```python
from build123d import *

# Parameters (mm, degrees)
F0_W      = 14.8
F0_H      = 16.7
F0_W_2    = 11.8
F0_H_2    = 13.7
F1_DEPTH  = 11.95
F2_W      = 12.65
F2_H      = 16.7
F2_W_2    = 10.65
F2_H_2    = 14.7
F3_DEPTH  = 7
F4_W      = 0.575
F4_H      = 13.7
F5_DEPTH  = 11.95
F6_W      = 0.575
F6_H      = 13.7
F7_DEPTH  = 11.95
F8_W      = 10.65
F8_H      = 0.5
F9_DEPTH  = 7
F10_W     = 10.65
F10_H     = 0.5
F11_DEPTH = 7
F12_W     = 14.8
F12_H     = 18.85
F12_W_2   = 10.65
F12_H_2   = 13.7
F13_DEPTH = 4.75


with BuildPart() as f1:
    # F0 (on Top) → F1 (new body)
    with BuildSketch(Plane.XY):
        Rectangle(F0_W, F0_H)
        Rectangle(F0_W_2, F0_H_2, mode=Mode.SUBTRACT)
    extrude(amount=F1_DEPTH)

    # F2 (on face) → F3 (join)
    with BuildSketch(Plane.XY.offset(11.95)):
        Rectangle(F2_W, F2_H)
        Rectangle(F2_W_2, F2_H_2, mode=Mode.SUBTRACT)
    extrude(amount=F3_DEPTH)

    # F4 (on face) → F5 (join, through all)
    with BuildSketch(Plane(origin=(0, 0, 11.95), x_dir=(1, 0, 0), z_dir=(0, 0, -1))):
        with Locations((-5.6125, 0)):
            Rectangle(F4_W, F4_H)
    extrude(amount=F5_DEPTH)

    # F6 (on face) → F7 (join, through all)
    with BuildSketch(Plane(origin=(0, 0, 11.95), x_dir=(1, 0, 0), z_dir=(0, 0, -1))):
        with Locations((5.6125, 0)):
            Rectangle(F6_W, F6_H)
    extrude(amount=F7_DEPTH)

    # F8 (on face) → F9 (join, through all)
    with BuildSketch(Plane.XY.offset(11.95)):
        with Locations((0, 7.1)):
            Rectangle(F8_W, F8_H)
    extrude(amount=F9_DEPTH)

    # F10 (on face) → F11 (join, through all)
    with BuildSketch(Plane.XY.offset(11.95)):
        with Locations((0, -7.1)):
            Rectangle(F10_W, F10_H)
    extrude(amount=F11_DEPTH)

    # F12 (on face) → F13 (join)
    with BuildSketch(Plane(origin=(0, 0, 0), x_dir=(1, 0, 0), z_dir=(0, 0, -1))):
        with Locations((0, -1.075)):
            Rectangle(F12_W, F12_H)
        Rectangle(F12_W_2, F12_H_2, mode=Mode.SUBTRACT)
    extrude(amount=F13_DEPTH)


solid = f1.part
```
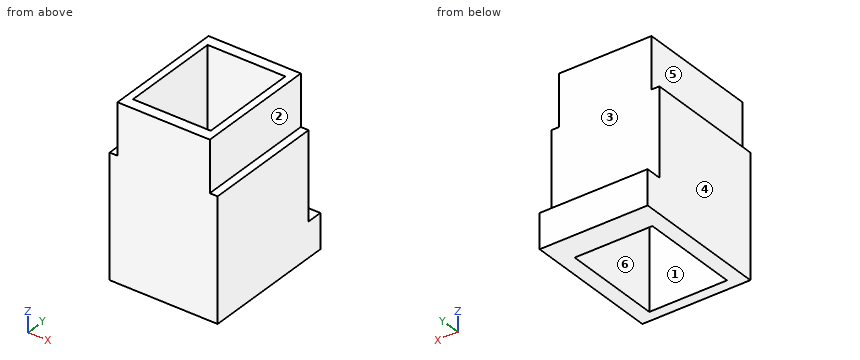
Input: part model. Units: mm. Frame: model coordinates. Face numbers are marked on the shaded views. A direction names the side the tool comes from. Round coordinates to 2 decimals unless told otherwise and drop trailing zeros. Loops run counter-clockwise (first coordinate to the right, second up) from the corner with the lowest first, then second, coordinate; pieces in that order, holes last. Notation, with made-up numbers: M 2.5,-25 L 27.5,-25 A31 cw 27.5,12 Z; hole C 12.5,5.5 d5. An arc over 180 degrees is marked long. Answer in a Markdown table with one row per item. Add a question column.
1. Contact query for flat-ended pins moving along their axis: pin 1 (1.2 mm diameter, centred on x = -7, y = 2.5, fed in from +Z); pin 2 (4 mm diameter, centred on x = -1, z = 6, fed in from +Y); pin 3 (2 mm diameter, centred on y = -1.5, z = 16, fed in from +X) (3 decimals). Output: stop coordinate, or through.
2. Ray query, probe 1 along Y at (x, z) = (2, 18); probe 2 along X at (y, z) = (-0.75, 3.5) (3 decimals); probe 3 along Y at (x, z) = (0.25, -2.25). Return the intervals inside material, ascending.
3. Section A-A (y = -1.5). Output: boundary loops of the cut face in (x, z) (3 decimals).
4. Set-up query: the marked faces 4, 5 and 6. Return all of +Z, -Z, +X, -X, +Y, -Y with unobstructed straight access to the full face (end or side cutting, diameter ignored); none if empty.
5. Section C-C (x = -4.75). Output: boundary loops of the cut face in (y, z).
6. Mould query, pull axis Y, two halves, no side actions, for the marked faces 1, 2 and 3. Classes: released by +Y, released by -Y, zero draft, split by the parting line, or undercut.
7. Section B-B (z = -3.5). Output: boundary loops of the cut face in (x, y) (3 decimals).
8. Section D-D (x = 5.75). Output: boundary loops of the cut face in (y, z), and give its area (3 significant figures).
Values follow:
| question | item | result |
|---|---|---|
| 1 | pin 1 | z = 11.95 |
| 1 | pin 2 | y = 8.35 |
| 1 | pin 3 | x = 6.325 |
| 2 | probe 1 | -8.35 to -6.85, 6.85 to 8.35 |
| 2 | probe 2 | -7.4 to -5.325, 5.325 to 7.4 |
| 2 | probe 3 | -8.35 to -6.85, 6.85 to 10.5 |
| 3 | outline | M -7.4,-4.75 L -5.325,-4.75 L -5.325,18.95 L -6.325,18.95 L -6.325,11.95 L -7.4,11.95 Z; M 5.325,-4.75 L 7.4,-4.75 L 7.4,11.95 L 6.325,11.95 L 6.325,18.95 L 5.325,18.95 Z |
| 4 | face 4 | +Z, -Z, -X, +Y, -Y |
| 4 | face 5 | +Z, -X, +Y, -Y |
| 4 | face 6 | +Z, -Z |
| 5 | outline | M -8.35,-4.75 L -6.85,-4.75 L -6.85,18.95 L -8.35,18.95 Z; M 6.85,-4.75 L 10.5,-4.75 L 10.5,0 L 8.35,0 L 8.35,18.95 L 6.85,18.95 Z |
| 6 | face 1 | undercut |
| 6 | face 2 | zero draft |
| 6 | face 3 | released by +Y |
| 7 | outline | M -7.4,-8.35 L 7.4,-8.35 L 7.4,10.5 L -7.4,10.5 Z; hole M -5.325,-6.85 L 5.325,-6.85 L 5.325,6.85 L -5.325,6.85 Z |
| 8 | outline | M -8.35,-4.75 L 10.5,-4.75 L 10.5,0 L 8.35,0 L 8.35,18.95 L -8.35,18.95 Z |
| 8 | area | 406 mm^2 |
